Model file for the job. Use its own axes, mm. Face numbers are marked on the shaded views. Round coordinates to 2 decimals unless told otherwise and drop trailing zeros. Write each loop counter-clockwise with the first axis right and the second up, starting at its lowest first coordinate (ties: lowest second). Pieces come first, ordered by that corner, then holes.
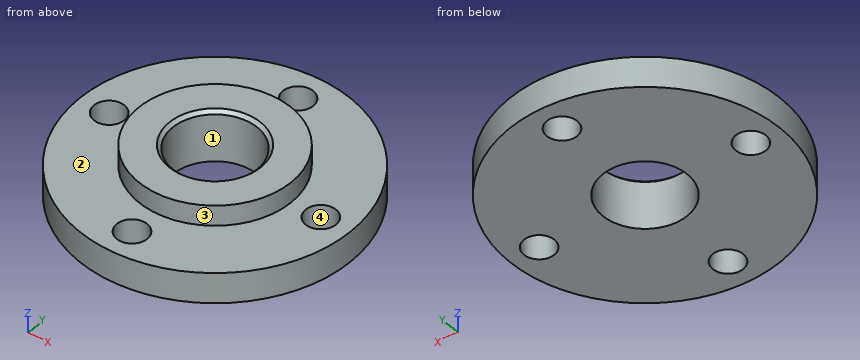
```python
from build123d import *

# Parameters (mm, degrees)
SKETCH_1_R          = 80
EXTRUDE_1_DEPTH     = 18
SKETCH_2_R          = 45
EXTRUDE_2_DEPTH     = 30
SKETCH_3_R          = 25
CUT_EXTRUDE_1_DEPTH = 118.046999107
SKETCH_4_R          = 9
CUT_EXTRUDE_2_DEPTH = 118.046999107
CHAMFER_1_SIZE      = 2


with BuildPart() as part:
    # 草图1 → 凸台-拉伸1 (new body)
    with BuildSketch(Plane.XY):
        Circle(SKETCH_1_R)
    extrude(amount=EXTRUDE_1_DEPTH)

    # 草图2 → 凸台-拉伸2 (add)
    with BuildSketch(Plane.XY):
        Circle(SKETCH_2_R)
    extrude(amount=EXTRUDE_2_DEPTH)

    # 草图3 → 切除-拉伸1 (cut, through all)
    with BuildSketch(Plane.XY):
        Circle(SKETCH_3_R)
    extrude(amount=CUT_EXTRUDE_1_DEPTH, mode=Mode.SUBTRACT)

    # 草图4 → 切除-拉伸2 (cut, through all)
    with BuildSketch(Plane.XY):
        with Locations((62.5, 0)):
            Circle(SKETCH_4_R)
        with Locations((0, 62.5)):
            Circle(SKETCH_4_R)
        with Locations((-62.5, 0)):
            Circle(SKETCH_4_R)
        with Locations((0, -62.5)):
            Circle(SKETCH_4_R)
    extrude(amount=CUT_EXTRUDE_2_DEPTH, mode=Mode.SUBTRACT)

    # 倒角1
    chamfer_1_edges = [part.edges().sort_by_distance(p)[0] for p in [
        (-25, 0, 30),
    ]]
    chamfer(chamfer_1_edges, length=CHAMFER_1_SIZE)


solid = part.part
```
1) Flat gauge pins, fed straight in: pin 1 Ø4 at (y, z) = (36, 6) entering from -X; pin 2 Ø1.5 at (x, y) = (-61.5, 9) entering from +Z; pin 3 Ø11 at (x, y) = (62.5, 0) entering from +Z; pin 4 Ø5 at (y, z) = (-58, 17) entering from -X. Where does each tip first touch, or does it go through?
2) Cut at A-A on y = 0. List the corners of the cut face in (x, z), and give its area (3 significant figures).
3) Wall check: probe 1 along Y at (x, z) = (0, 9.25); probe 2 along Z at (x, y) = (51, -10); probe 3 along Y at (x, z) = (-56, 8.5). Give the ranges that are in metal, low to high.
4) Pull direction X, two halves, no side cores. Call the marked faces 1, 2, 3 and 4: released by +X, released by -X, zero draft, split by the parting line, or undercut.
5) Cut at C-C on y = 68.5. List the corners of the cut face in (x, z).
6) Cut at D-D on z = 7.5. List the corners of the cut face in (x, y), and give its area (3 significant figures).
Result sheet:
1. pin 1: stops at x = -72.42
1. pin 2: stops at z = 18
1. pin 3: passes through
1. pin 4: stops at x = -57.62
2. outline: (-80, 0) - (-71.5, 0) - (-71.5, 18) - (-80, 18) - close; (-53.5, 0) - (-25, 0) - (-25, 28) - (-27, 30) - (-45, 30) - (-45, 18) - (-53.5, 18) - close; (25, 0) - (53.5, 0) - (53.5, 18) - (45, 18) - (45, 30) - (27, 30) - (25, 28) - close; (71.5, 0) - (80, 0) - (80, 18) - (71.5, 18) - close
2. area: 1,810 mm2
3. probe 1: y = -80 to -71.5, -53.5 to -25, 25 to 53.5, 71.5 to 80
3. probe 2: z = 0 to 18
3. probe 3: y = -57.13 to -6.22, 6.22 to 57.13
4. face 1: undercut
4. face 2: zero draft
4. face 3: split by the parting line
4. face 4: undercut
5. outline: (-41.32, 0) - (-6.71, 0) - (-6.71, 18) - (-41.32, 18) - close; (6.71, 0) - (41.32, 0) - (41.32, 18) - (6.71, 18) - close
6. outline: circle Ø160 at (0, 0); hole circle Ø18 at (-62.5, 0); hole circle Ø50 at (0, 0); hole circle Ø18 at (0, -62.5); hole circle Ø18 at (0, 62.5); hole circle Ø18 at (62.5, 0)
6. area: 17,100 mm2
